from build123d import *

# Parameters (mm, degrees)
CYLINDER003_R     = 6.2
CYLINDER003_DEPTH = 10
BOX006_W          = 45.1
BOX006_H          = 20
BOX006_DEPTH      = 2
BOX005_W          = 5
BOX005_H          = 5
BOX005_DEPTH      = 2
BOX004_W          = 5
BOX004_H          = 5
BOX004_DEPTH      = 2


with BuildPart() as cylinder:
    # Cylinder003 → Cylinder003 (new body)
    with BuildSketch(Plane(origin=(62.15, 0, -10), x_dir=(1, 0, 0), z_dir=(0, 0, 1))):
        Circle(CYLINDER003_R)
    extrude(amount=CYLINDER003_DEPTH)


with BuildPart() as cube003:
    # Box006 → Box006 (new body)
    with BuildSketch(Plane(origin=(47.5, -10, -2), x_dir=(1, 0, 0), z_dir=(0, 0, 1))):
        with Locations((22.55, 10)):
            Rectangle(BOX006_W, BOX006_H)
    extrude(amount=BOX006_DEPTH)


with BuildPart() as cube002:
    # Box005 → Box005 (new body)
    with BuildSketch(Plane(origin=(59.5, 10, -2), x_dir=(1, 0, 0), z_dir=(0, 0, 1))):
        with Locations((2.5, 2.5)):
            Rectangle(BOX005_W, BOX005_H)
    extrude(amount=BOX005_DEPTH)


with BuildPart() as obj1:
    # Box004 → Box004 (new body)
    with BuildSketch(Plane(origin=(59.5, -15, -2), x_dir=(1, 0, 0), z_dir=(0, 0, 1))):
        with Locations((2.5, 2.5)):
            Rectangle(BOX004_W, BOX004_H)
    extrude(amount=BOX004_DEPTH)

    # Fusion004: union Cube002
    add(cube002.part)

    # Fusion005: union Cube003
    add(cube003.part)

    # Fusion006: union Cylinder
    add(cylinder.part)


solid = obj1.part
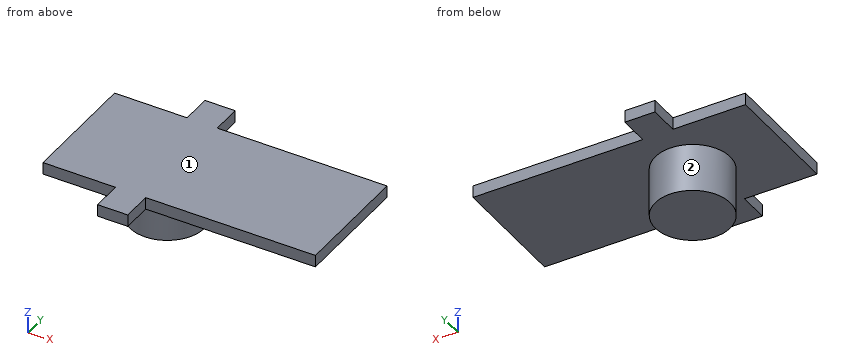
The model under review builds one solid part; all positions refer to its coordinate system, in mm. Face numbers are marked on the shaded views. A direction names the side the tool comes from. Coordinates: 2 decimals unless noted, no trailing zeros. Loops run counter-clockwise (first coordinate to the right, second up) from the corner with the lowest first, then second, coordinate; pieces in that order, holes last.
(1) Consider section A-A, the plane z = -1.25. Give the boundary of the cut face in (x, y).
Determined:
outline: (47.5, -10) - (59.5, -10) - (59.5, -15) - (64.5, -15) - (64.5, -10) - (92.6, -10) - (92.6, 10) - (64.5, 10) - (64.5, 15) - (59.5, 15) - (59.5, 10) - (47.5, 10) - close
(2) Consider section D-D, the plane x = 80. Give the boundary of the cut face in (y, z), plus the area to 3 significant figures.
Determined:
outline: (-10, -2) - (10, -2) - (10, 0) - (-10, 0) - close
area: 40.0 mm2
(3) Consider section C-C, the plane y = 0. Give the boundary of the cut face in (x, z).
Determined:
outline: (47.5, -2) - (55.95, -2) - (55.95, -10) - (68.35, -10) - (68.35, -2) - (92.6, -2) - (92.6, 0) - (47.5, 0) - close
(4) Wall thickness on L1, parallel to Z at x = 87, y = -5; L2, parallel to Y at x = 69.5, z = -1.5; L3, parallel to X at y = 4.5, z = -7: over which ranges is each line inside the solid? List them lowest first.
Determined:
L1: z = -2 to 0
L2: y = -10 to 10
L3: x = 57.89 to 66.41
(5) Insertion check: P1, Ø2, axis at y = 11.5, z = -1, coming from the -X side; P2, Ø1, axis at y = 12.5, z = -1, coming from the +X side; P3, Ø3, axis at x = 74, z = -1.5, coming from the -Y side; P4, Ø4, axis at x = 75.5, z = -5, coming from the -Y side. Each pin has a flat end and moves straight along its axis. Give the tip position at first contact, or say it passes through.
Determined:
P1: stops at x = 59.5
P2: stops at x = 64.5
P3: stops at y = -10
P4: passes through
(6) Consider section B-B, the plane x = 62.15. Give the boundary of the cut face in (y, z).
Determined:
outline: (-15, -2) - (-6.2, -2) - (-6.2, -10) - (6.2, -10) - (6.2, -2) - (15, -2) - (15, 0) - (-15, 0) - close
(7) Tool access review of the marked faces 1 and 2: name each direction out of +Z, -Z, +X, -X, +Y, -Y from which nothing blocks a thin tool from reaching the whole face with its end or side.
Determined:
face 1: +Z, +X, -X, +Y, -Y
face 2: -Z
